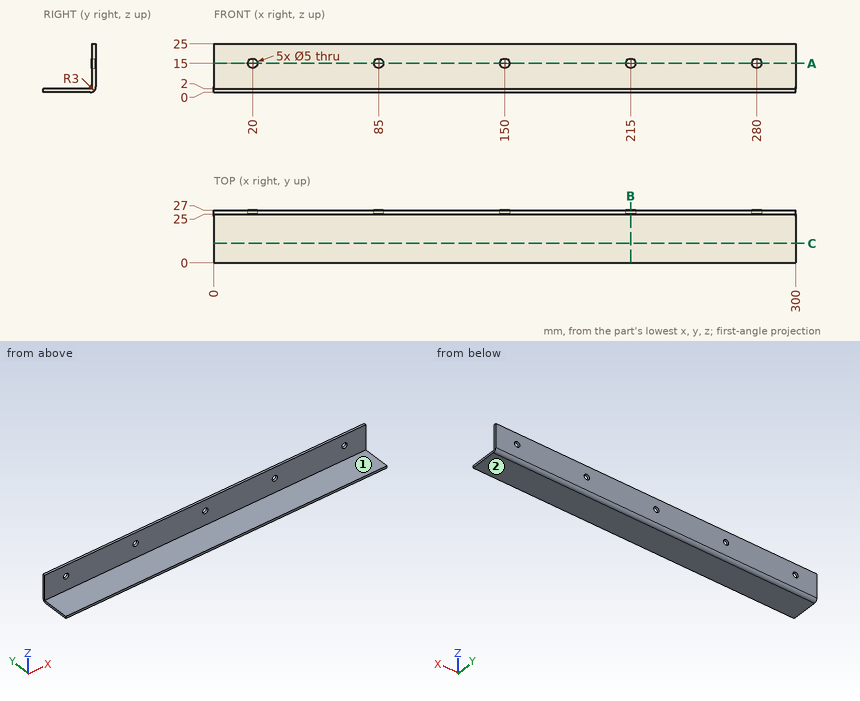
The figure shows three views and two pictorial views of one solid part (mm, origin at its lowest corner). Answer the questions. A direction names the side the tool comes from. Give positions to 0.01 mm unless a question says otherwise; leave off trailing zeros. Write each loop counter-clockwise with the first axis right and the second up, starting at its lowest first coordinate (ties: lowest second). Pieces come first, ordered by that corner, then holes.
Q1. A tool of negligible diameter and unlimited length cuts with its end or side. For the marked faces 1 and 2, from which of +Z, -Z, +X, -X, +Y, -Y can it reach the whole face along a straight path? Write none if from no direction.
Answer:
face 1: +Z, +X, -X, -Y
face 2: -Z, +X, -X, +Y, -Y
Q2. Straight lines are drawn through the part: L1, parallel to X at y = 26.1, z = 15; L2, parallel to Y at x = 114, z = 15.75; L3, parallel to Z at x = 81, y = 10.25. For each, find the intervals that lie inside material, in ascending order.
Answer:
L1: x = 0 to 17.5, 22.5 to 82.5, 87.5 to 147.5, 152.5 to 212.5, 217.5 to 277.5, 282.5 to 300
L2: y = 25 to 27
L3: z = 0 to 2
Q3. The part is cut by section C-C on y = 10. Give the vertices of the cut face in (x, z).
Answer:
outline: (0, 0) - (300, 0) - (300, 2) - (0, 2) - close
Q4. Given pin 1 (2 mm diameter, centred on x = 109, y = 22.5, fed in from +Z); pin 2 (6 mm diameter, centred on x = 215, z = 15, fed in from -Y), each flat-ended and moving along its own axis, determine where each tip first touches the part or whether it passes through.
Answer:
pin 1: stops at z = 2
pin 2: stops at y = 25
Q5. The part is cut by section B-B on x = 215. Give the vertices of the cut face in (y, z), and give its area (3 significant figures).
Answer:
outline: (0, 0) - (24, 0) arc R3 ccw to (27, 3) - (27, 12.5) - (25, 12.5) - (25, 2) - (0, 2) - close; (25, 17.5) - (27, 17.5) - (27, 25) - (25, 25) - close
area: 88.1 mm2
Q6. The part is cut by section A-A on z = 15. Give the vertices of the cut face in (x, y).
Answer:
outline: (0, 25) - (17.5, 25) - (17.5, 27) - (0, 27) - close; (22.5, 25) - (82.5, 25) - (82.5, 27) - (22.5, 27) - close; (87.5, 25) - (147.5, 25) - (147.5, 27) - (87.5, 27) - close; (152.5, 25) - (212.5, 25) - (212.5, 27) - (152.5, 27) - close; (217.5, 25) - (277.5, 25) - (277.5, 27) - (217.5, 27) - close; (282.5, 25) - (300, 25) - (300, 27) - (282.5, 27) - close
